from build123d import *

# Parameters (mm, degrees)
SKETCH1_W           = 88.9
SKETCH1_H           = 76.2
BOSS_EXTRUDE1_DEPTH = 19.05
SKETCH2_R           = 3.175
CUT_EXTRUDE1_DEPTH  = 12.7


with BuildPart() as part:
    # Sketch1 → Boss-Extrude1 (new body)
    with BuildSketch(Plane(origin=(0, 0, 0), x_dir=(1, 0, 0), z_dir=(0, 1, 0))):
        Rectangle(SKETCH1_W, SKETCH1_H)
    extrude(amount=BOSS_EXTRUDE1_DEPTH)

    # Sketch2 → Cut-Extrude1 (cut)
    with BuildSketch(Plane.XY.offset(38.1)):
        with Locations((-12.7, 9.525)):
            Circle(SKETCH2_R)
        with Locations((12.7, 9.525)):
            Circle(SKETCH2_R)
    extrude(amount=-CUT_EXTRUDE1_DEPTH, mode=Mode.SUBTRACT)


solid = part.part
Model file for the job. Use its own axes, mm. A direction names the side the tool comes from. Give positions to 0.01 mm unless a question says otherwise; leave off trailing zeros. Order: outer loops, then holes, each group sorted by start corner. A loop starts at its lowest first (then second) coordinate and runs counter-clockwise, first axis right, second up. Notation, with made-up numbers: M -7.75,-16 L 22.25,-16 A37 ccw 22.25,23 Z; hole C -3,37.5 d11. An arc over 180 degrees is marked long. Write item = value, one per line.
Q1. Cut at A-A, the plane x = -12.7. List the corners of the cut face in (y, z).
Derived:
outline = M 0,-38.1 L 19.05,-38.1 L 19.05,38.1 L 12.7,38.1 L 12.7,25.4 L 6.35,25.4 L 6.35,38.1 L 0,38.1 Z
Q2. Flat gauge pin, fed straight in: pin 1 (1.9 mm diameter, centred on x = -11.5, y = 8, fed in from +Z). Where does the tip first touch, or does it go through?
Derived:
pin_1 = 25.4
Q3. Cut at B-B, the plane x = 13. List the corners of the cut face in (y, z), then the cut area to 3 significant figures.
Derived:
outline = M 0,-38.1 L 19.05,-38.1 L 19.05,38.1 L 12.69,38.1 L 12.69,25.4 L 6.36,25.4 L 6.36,38.1 L 0,38.1 Z
area = 1,370 mm2
Q4. Two-plate mould, pull along Y, no slides. Class faces 3 (the flat face through (-1, 0, -1)), 4 (the flat face through (-1, 9, -38.1)), 5 (the cylindrical face through (-10.99, 12.2, 31.84)): pulls with the +Y half, pulls with the -Y half, needs draft (parallel to the pull), parting line crosses it, or undercut.
Derived:
face_3 = pulls with the -Y half
face_4 = needs draft
face_5 = undercut
Q5. Tool access for faces 1 (the cylindrical face through (10.36, 11.67, 31.84)), 2 (the flat face through (-1, 19.05, -1)): list every direction of +Z, -Z, +X, -X, +Y, -Y with a clear straight run to the whole face (end or side of a thin tool).
Derived:
face_1 = +Z
face_2 = +Z, -Z, +X, -X, +Y
Q6. Drill centre lines: line 1 (Y direction, x = -12.7, z = 31.75); line 2 (Z direction, x = -11, y = 7); line 3 (Y direction, x = 12, z = 35). Where is each one in solid material? Low to high. Write a range as [from, to].
Derived:
line_1 = [0, 6.35], [12.7, 19.05]
line_2 = [-38.1, 25.4]
line_3 = [0, 6.43], [12.62, 19.05]
